Input: dimensioned drawing with shaded views. Units: mm. Origin: part minimum x, y, z. A direction names the side the tool comes from. Coordinates: 2 decimals unless noted, no trailing zeros. Order: outer loops, then holes, each group sorted by start corner. A loop starts at its lowest first (then second) coordinate and runs counter-clockwise, first axis right, second up. Notation, with made-up numbers: (-20, 18) -> (37, 18) arc R25 ccw to (37, 46) -> close; hole circle Ø6 at (33.25, 17). An arc over 180 degrees is marked (long way). Put each result on its own line as item: value.
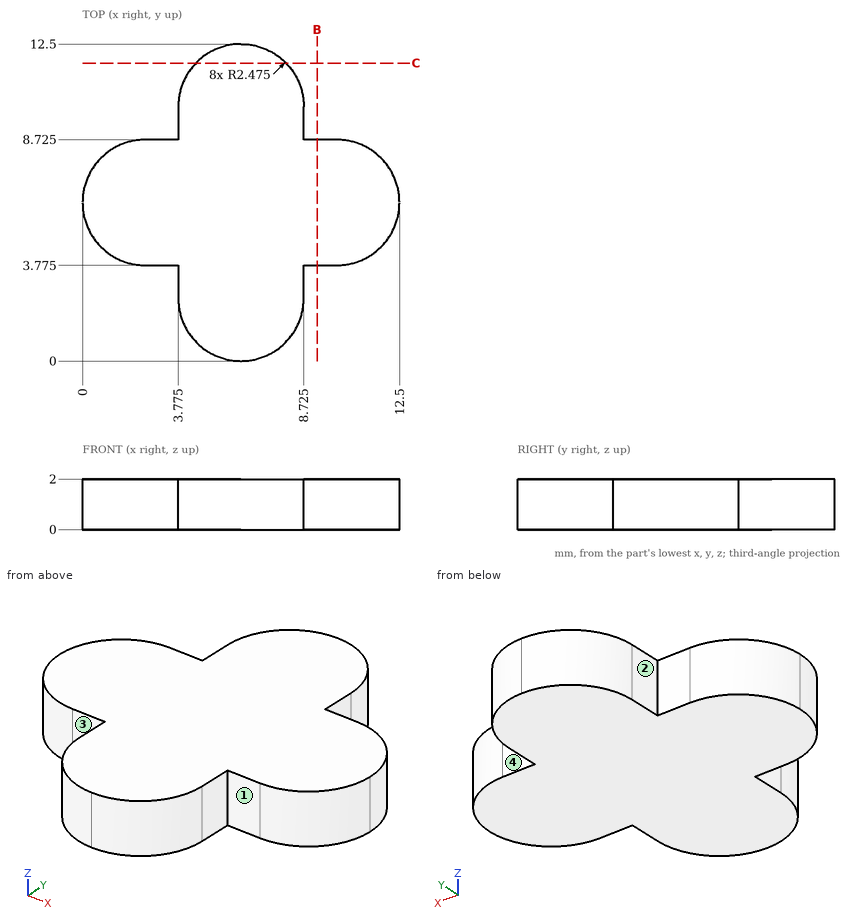
1. Set-up query: the marked faces 1, 2, 3 and 4. Return all of +Z, -Z, +X, -X, +Y, -Y with unobstructed straight access to the full face (end or side cutting, diameter ignored); none if empty.
Numbers:
face 1: +Z, -Z, +X, -Y
face 2: +Z, -Z, -X, +Y
face 3: +Z, -Z, -X, -Y
face 4: +Z, -Z, +X, +Y
2. Ray query, line 1 along Y through (x, z) = (9, 1.5) (3 decimals); line 2 along Y through (x, z) = (10.75, 1.2). Return the intervals inside material, ascending.
Numbers:
line 1: y = 3.775 to 8.725
line 2: y = 3.88 to 8.62
3. Cut plane C-C on y = 11.75. Output: boundary loops of the cut face in (x, z) (3 decimals), plus the area to 3 significant figures.
Numbers:
outline: (4.475, 0) -> (8.025, 0) -> (8.025, 2) -> (4.475, 2) -> close
area: 7.10 mm2
4. Cut plane B-B on x = 9.25. Output: boundary loops of the cut face in (y, z) (3 decimals), plus the area to 3 significant figures.
Numbers:
outline: (3.775, 0) -> (8.725, 0) -> (8.725, 2) -> (3.775, 2) -> close
area: 9.90 mm2
5. First-contact query: pin 1 (1 mm diameter, centred on x = 2, z = 0.5, fed in from -Y) (3 decimals); pin 2 (0.7 mm diameter, centred on y = 9.5, z = 1, fed in from +X) (3 decimals); pin 3 (0.7 mm diameter, centred on y = 3, z = 1.5, fed in from -X) (3 decimals). Flat tips, straight axial feed; report the tip coordinate or a pass-through.
Numbers:
pin 1: stops at y = 3.775
pin 2: stops at x = 8.725
pin 3: stops at x = 3.775
